from build123d import *

# Parameters (mm, degrees)
EXTRUDE_1_DEPTH = 1.5
SKETCH_2_W      = 18
SKETCH_2_H      = 17.9
EXTRUDE_2_DEPTH = 0.5
SKETCH_3_W      = 18
SKETCH_3_H      = 1.2
EXTRUDE_3_DEPTH = 8


with BuildPart() as part:
    # 草图1 → 凸台-拉伸1 (new body)
    with BuildSketch(Plane(origin=(0, 0, 0), x_dir=(1, 0, 0), z_dir=(0, 1, 0))):
        Polygon((18, 10.1), (18, 17.9), (0, 17.9), (0, 0), (18, 0), (18, 7.8), (38, 7.8), (38, 10.1), align=None)
    extrude(amount=EXTRUDE_1_DEPTH)

    # 草图2 → 凸台-拉伸2 (add)
    with BuildSketch(Plane(origin=(0, 1.5, 0), x_dir=(1, 0, 0), z_dir=(0, 1, 0))):
        with Locations((9, 8.95)):
            Rectangle(SKETCH_2_W, SKETCH_2_H)
    extrude(amount=EXTRUDE_2_DEPTH)

    # 草图3 → 凸台-拉伸3 (add)
    with BuildSketch(Plane(origin=(0, 2, 0), x_dir=(1, 0, 0), z_dir=(0, 1, 0))):
        with Locations((9, 17.3)):
            Rectangle(SKETCH_3_W, SKETCH_3_H)
        with Locations((9, 0.6)):
            Rectangle(SKETCH_3_W, SKETCH_3_H)
    extrude(amount=EXTRUDE_3_DEPTH)


solid = part.part
Verification items for the finished model (mm, model axes). A direction names the side the tool comes from. Round coordinates to 2 decimals unless told otherwise and drop trailing zeros. Loops run counter-clockwise (first coordinate to the right, second up) from the corner with the lowest first, then second, coordinate; pieces in that order, holes last. Notation, with made-up numbers: (-6.75, 32) - (26.25, 32) arc R29 ccw to (26.25, 69) - close; hole circle Ø8 at (39.25, -8.5). An arc over 180 degrees is marked (long way). Answer in a Markdown table with one row per item. Add a question column.
Q1. Section check C-C on y = 0.5. Enter the section's corners in (x, z), plus the area to 3 significant figures.
Q2. Section check A-A on y = 8. Enter the section's corners in (x, z), plus the area to 3 significant figures.
Q3. Release check for a two-part mould opening along Z. For faces 5 (the face through (9, 5, -17.9)), 6 (the face through (9, 10, -1)), 7 (the face through (9, 2, -9)) record: pulls with the +Z half, pulls with the -Z half, needs draft (parallel to the pull), parting line crosses it, or undercut.
Q4. Gauge pin test, flat ends, axial feed: pin 1 (5 mm diameter, centred on y = 4, z = -5.5, fed in from +X); pin 2 (1.2 mm diameter, centred on x = 23, y = 0.5, fed in from -Z); pin 3 (0.7 mm diameter, centred on x = 32.5, z = -8.5, fed in from +Y). Record the tip position at first contact, or that the pin passes through.
Q5. Section check D-D on z = -8.5. Enter the section's corners in (x, y).
Q6. Tool access check on faces 1 (the face through (28, 1, -10.1)), 2 (the face through (9, 6, -16.7)), 3 (the face through (28, 1.5, -9)), 4 (the face through (28, 1, -7.8)). Record the directions out of +Z, -Z, +X, -X, +Y, -Y that give a thin tool (end or side, any length) a straight path to the whole face; none if there is none.
Q7. Section check B-B on x = 11. Enter the section's corners in (y, z).
Q8. Material ranges on line 1 (Z direction, x = 10, y = 5.5); line 2 (X direction, y = 1, z = -3.5); line 3 (Y direction, x = 13, z = -1.75), recorded low to high.
Found:
| question | item | result |
|---|---|---|
| 1 | outline | (0, -17.9) - (18, -17.9) - (18, -10.1) - (38, -10.1) - (38, -7.8) - (18, -7.8) - (18, 0) - (0, 0) - close |
| 1 | area | 368 mm² |
| 2 | outline | (0, -17.9) - (18, -17.9) - (18, -16.7) - (0, -16.7) - close; (0, -1.2) - (18, -1.2) - (18, 0) - (0, 0) - close |
| 2 | area | 43.2 mm² |
| 3 | face 5 | pulls with the -Z half |
| 3 | face 6 | needs draft |
| 3 | face 7 | undercut |
| 4 | pin 1 | stops at x = 18 |
| 4 | pin 2 | stops at z = -10.1 |
| 4 | pin 3 | stops at y = 1.5 |
| 5 | outline | (0, 0) - (38, 0) - (38, 1.5) - (18, 1.5) - (18, 2) - (0, 2) - close |
| 6 | face 1 | -Z, +X, +Y, -Y |
| 6 | face 2 | +X, -X, +Y |
| 6 | face 3 | +Z, -Z, +X, +Y |
| 6 | face 4 | +Z, +X, +Y, -Y |
| 7 | outline | (0, -17.9) - (10, -17.9) - (10, -16.7) - (2, -16.7) - (2, -1.2) - (10, -1.2) - (10, 0) - (0, 0) - close |
| 8 | line 1 | z = -17.9 to -16.7, -1.2 to 0 |
| 8 | line 2 | x = 0 to 18 |
| 8 | line 3 | y = 0 to 2 |
